from build123d import *

# Parameters (mm, degrees)
SKIZZE1_R                                 = 11.5
GRUNDK_RPER_WALZE_DEPTH                   = 74
PRESSPASSUNG_KUGELLAGER_DEPTH             = 4.3
SKIZZE3_R                                 = 2.25
M4_SCHRAUBENF_HRUNG_DEPTH                 = 4.5
SKIZZE4_R                                 = 9.6
MOTORAUSSPARUNG_DEPTH                     = 12.75
ZERST_RUNGSELEMENT_START                  = -6
SKIZZE7_W                                 = 1.5
SKIZZE7_H                                 = 15
ZERST_RUNGSELEMENT_AUSSPARUNG_DEPTH       = 63
SKIZZE8_W                                 = 63
SKIZZE8_H                                 = 4
ZERST_RUNGSELEMENT_RECHTECK_DEPTH         = 1.5
M5_MOTOR_MUTTER_DEPTH                     = 12
SKIZZE12_R                                = 3.1
M5_AUSLAUF_SCHRAUBE_DEPTH                 = 2
ZERST_RUNGSELEMENT_VERVIELF_LTIGUNG_COUNT = 3
SKIZZE13_R                                = 8.5
INNENAUSPARUNG_HOHL_DEPTH                 = 38


with BuildPart() as part:
    # Skizze1 → Grundkörper Walze (new body)
    with BuildSketch(Plane(origin=(0, 0, 0), x_dir=(0, 0, -1), z_dir=(1, 0, 0))):
        Circle(SKIZZE1_R)
    extrude(amount=GRUNDK_RPER_WALZE_DEPTH)

    # Skizze2 → Presspassung Kugellager (cut)
    with BuildSketch(Plane(origin=(74, 0, 0), x_dir=(0, 0, -1), z_dir=(1, 0, 0))):
        with BuildLine():
            Line((-7.040453047, 1.507322425), (-6.940453047, 1.507322425))
            Line((-6.940453047, 1.507322425), (-6.940453047, -1.492677575))
            Line((-6.940453047, -1.492677575), (-7.043572507, -1.492677575))
            ThreePointArc((-7.043572507, -1.492677575), (-5.829319782, -4.225994662), (-3.609168454, -6.230080503))
            Line((-3.609168454, -6.230080503), (-3.578266755, -6.134974851))
            Line((-3.578266755, -6.134974851), (-0.725097206, -7.062025834))
            Line((-0.725097206, -7.062025834), (-0.756962871, -7.160098268))
            ThreePointArc((-0.756962871, -7.160098268), (2.217800882, -6.849916733), (4.809864271, -5.357723928))
            Line((4.809864271, -5.357723928), (4.728962572, -5.298945403))
            Line((4.728962572, -5.298945403), (6.492318329, -2.87189442))
            Line((6.492318329, -2.87189442), (6.575743724, -2.932506518))
            ThreePointArc((6.575743724, -2.932506518), (7.199996108, -0.007486699), (6.581828055, 2.918825013))
            Line((6.581828055, 2.918825013), (6.500926356, 2.860046487))
            Line((6.500926356, 2.860046487), (4.737570599, 5.28709747))
            Line((4.737570599, 5.28709747), (4.820995994, 5.347709568))
            ThreePointArc((4.820995994, 5.347709568), (2.232041431, 6.845289698), (-0.742070825, 7.161656993))
            Line((-0.742070825, 7.161656993), (-0.711169126, 7.066551342))
            Line((-0.711169126, 7.066551342), (-3.564338674, 6.139500359))
            Line((-3.564338674, 6.139500359), (-3.59620434, 6.237572793))
            ThreePointArc((-3.59620434, 6.237572793), (-5.820518639, 4.238108396), (-7.040453047, 1.507322425))
        make_face()
    extrude(amount=-PRESSPASSUNG_KUGELLAGER_DEPTH, mode=Mode.SUBTRACT)

    # Skizze3 → M4 Schraubenführung (cut)
    with BuildSketch(Plane(origin=(69.7, 0, 0), x_dir=(0, 0, -1), z_dir=(1, 0, 0))):
        Circle(SKIZZE3_R)
    extrude(amount=-M4_SCHRAUBENF_HRUNG_DEPTH, mode=Mode.SUBTRACT)

    # Skizze4 → Motoraussparung (cut)
    with BuildSketch(Plane.ZY):
        Circle(SKIZZE4_R)
    extrude(amount=-MOTORAUSSPARUNG_DEPTH, mode=Mode.SUBTRACT)

    # Skizze7 → Zerstörungselement Aussparung (cut)
    with BuildSketch(Plane(origin=(74, 0, 0), x_dir=(0, 0, -1), z_dir=(1, 0, 0)).offset(ZERST_RUNGSELEMENT_START)):
        with Locations((-10.75, 0)):
            Rectangle(SKIZZE7_W, SKIZZE7_H)
    zerst_rungselement_aussparung = extrude(amount=-ZERST_RUNGSELEMENT_AUSSPARUNG_DEPTH, mode=Mode.SUBTRACT)

    # Skizze8 → Zerstörungselement Rechteck (add)
    with BuildSketch(Plane.XY.offset(10)):
        with Locations((36.5, 0)):
            Rectangle(SKIZZE8_W, SKIZZE8_H)
    zerst_rungselement_rechteck = extrude(amount=ZERST_RUNGSELEMENT_RECHTECK_DEPTH)

    # Skizze10 → M5 Motor Mutter (cut)
    with BuildSketch(Plane.ZY.offset(-12.75)):
        Polygon((4.139835299, -2.29675794), (4.058968371, 2.436823566), (-0.080866927, 4.733581506), (-4.139835299, 2.29675794), (-4.058968371, -2.436823566), (0.080866927, -4.733581506), align=None)
    extrude(amount=-M5_MOTOR_MUTTER_DEPTH, mode=Mode.SUBTRACT)

    # Skizze12 → M5 Auslauf Schraube (cut)
    with BuildSketch(Plane.ZY.offset(-24.75)):
        Circle(SKIZZE12_R)
    extrude(amount=-M5_AUSLAUF_SCHRAUBE_DEPTH, mode=Mode.SUBTRACT)

    # Zerstörungselement Vervielfältigung: Zerstörungselement Aussparung, Zerstörungselement Rechteck ×3 about axis
    zerst_rungselement_vervielf_ltigung_axis = Axis((0, 0, 0), (1, 0, 0))
    add([zerst_rungselement_aussparung.rotate(zerst_rungselement_vervielf_ltigung_axis, i * 360 / ZERST_RUNGSELEMENT_VERVIELF_LTIGUNG_COUNT) for i in range(1, ZERST_RUNGSELEMENT_VERVIELF_LTIGUNG_COUNT)], mode=Mode.SUBTRACT)
    add([zerst_rungselement_rechteck.rotate(zerst_rungselement_vervielf_ltigung_axis, i * 360 / ZERST_RUNGSELEMENT_VERVIELF_LTIGUNG_COUNT) for i in range(1, ZERST_RUNGSELEMENT_VERVIELF_LTIGUNG_COUNT)])

    # Skizze13 → Innenausparung hohl (cut)
    with BuildSketch(Plane(origin=(65.2, 0, 0), x_dir=(0, 0, -1), z_dir=(1, 0, 0))):
        Circle(SKIZZE13_R)
    extrude(amount=-INNENAUSPARUNG_HOHL_DEPTH, mode=Mode.SUBTRACT)


solid = part.part
Could you check a few things on this model? Use its own coordinates, in mm. A direction names the side the tool comes from. Give positions to 0.01 mm unless a question says otherwise; leave off trailing zeros. Order: outer loops, then holes, each group sorted by start corner. A loop starts at its lowest first (then second) coordinate and runs counter-clockwise, first axis right, second up. Notation, with made-up numbers: (68, 40) - (112, 40) arc R32 ccw to (112, 67) - close; hole circle Ø9 at (20.5, -32). An arc over 180 degrees is marked (long way). Return JSON: item names as keys, results as strings. Group by question number.
Q1. Suppose I cut it at B-B, the plane x = 23.5. Please give me the cut outline in (y, z).
Q2. Thinking about a two-plate mould opening in Y: for faces 6 (the face through (36.941, -10.567, -1.697)), 7 (the face through (36.059, 10.301, -3.638)), 8 (the face through (68, -3.4, 10.5)), 9 (the face through (18.666, 3.532, -2.082)), which applies, pulls with the +Y half, pulls with the -Y half, needs draft (parallel to the pull), parting line crosses it, or undercut?
Q3. Suppose I cut it at A-A, the plane x = 56.5. Please give me the cut outline in (y, z), and give its area (3 significant figures).
Q4. Which directions (+Z, -Z, +X, -X, +Y, -Y) give clear straight access to the entire face, cutting with the end or side of a thin tool? Please do faces 1 (the face through (27.2, 0, 0)), 2 (the face through (18.67, -3.57, -2.02)), 3 (the face through (5, 3.5, 10.5)), 4 (the face through (68, 11, -2)), 5 (the face through (5, -11, -2)).
Q5. Please list where these lines run through material, in increasing order: line 1 along X through (y, z) = (-2.75, -5.5); line 2 along Y through (x, z) = (68.1, 0); line 3 along Y through (x, z) = (36, 0.25). Write a range as [from, to].
Q6. Will these pins go through, and if not, where does the flat tip stop? pin 1 Ø4 at (y, z) = (0, 0) entering from +X; pin 2 Ø4 at (x, y) = (33.5, -2.5) entering from -Z; pin 3 Ø10 at (x, z) = (53, 6.5) entering from +Y.
Resolved:
{
 "1": {"outline": "(-11.5, -0.08) - (-9.66, -3.27) - (-10.96, -4.02) - (-8.96, -7.48) - (-7.66, -6.73) - (-5.82, -9.92) arc R11.5 ccw to (5.82, -9.92) - (7.66, -6.73) - (8.96, -7.48) - (10.96, -4.02) - (9.66, -3.27) - (11.5, -0.08) arc R11.5 ccw to (5.68, 10) - (2, 10) - (2, 11.5) - (-2, 11.5) - (-2, 10) - (-5.68, 10) arc R11.5 ccw to start; hole (-4.73, 0.08) - (-2.44, -4.06) - (2.3, -4.14) - (4.73, -0.08) - (2.44, 4.06) - (-2.3, 4.14) - close"},
 "2": {"face 6": "pulls with the -Y half", "face 7": "pulls with the +Y half", "face 8": "needs draft", "face 9": "undercut"},
 "3": {"outline": "(-11.5, -0.08) - (-9.66, -3.27) - (-10.96, -4.02) - (-8.96, -7.48) - (-7.66, -6.73) - (-5.82, -9.92) arc R11.5 ccw to (5.82, -9.92) - (7.66, -6.73) - (8.96, -7.48) - (10.96, -4.02) - (9.66, -3.27) - (11.5, -0.08) arc R11.5 ccw to (5.68, 10) - (2, 10) - (2, 11.5) - (-2, 11.5) - (-2, 10) - (-5.68, 10) arc R11.5 ccw to start; hole circle Ø17 at (0, 0)", "area": "172 mm2"},
 "4": {"face 1": "none", "face 2": "-X", "face 3": "+Z, +Y", "face 4": "+Y", "face 5": "-Y"},
 "5": {"line 1": "x = [12.75, 27.2], [65.2, 69.7]", "line 2": "y = [-11.5, -2.25], [2.25, 11.5]", "line 3": "y = [-11.5, -8.5], [8.5, 11.5]"},
 "6": {"pin 1": "stops at x = 27.2", "pin 2": "stops at z = -11.49", "pin 3": "stops at y = 11.4"}
}
